```python
from build123d import *

# Parameters (mm, degrees)
SKETCH1_W                   = 355
SKETCH1_H                   = 210
BOSS_EXTRUDE1_DEPTH         = 6
SKETCH2_W                   = 355
SKETCH2_H                   = 92
BOSS_EXTRUDE2_DEPTH         = 7
M4_TAPPED_HOLE2_D           = 3.3
M4_TAPPED_HOLE2_DEPTH       = 2.008579979
M4_TAPPED_HOLE2_CSINK_D     = 4.05
M4_TAPPED_HOLE2_CSINK_ANGLE = 90
M4_TAPPED_HOLE2_TIP         = 0.991420021


with BuildPart() as part:
    # Sketch1 → Boss-Extrude1 (new body)
    with BuildSketch(Plane.XY):
        Rectangle(SKETCH1_W, SKETCH1_H)
    extrude(amount=BOSS_EXTRUDE1_DEPTH)

    # Sketch2 → Boss-Extrude2 (add)
    with BuildSketch(Plane.XY):
        with Locations((0, -59)):
            Rectangle(SKETCH2_W, SKETCH2_H)
    extrude(amount=-BOSS_EXTRUDE2_DEPTH)

    # M4 Tapped Hole2
    with Locations(Plane(origin=(0, 0, -7), x_dir=(-1, 0, 0), z_dir=(0, 0, -1))):
        with Locations((37.5, -29), (-37.5, -29)):
            CounterSinkHole(M4_TAPPED_HOLE2_D / 2, M4_TAPPED_HOLE2_CSINK_D / 2, depth=M4_TAPPED_HOLE2_DEPTH, counter_sink_angle=M4_TAPPED_HOLE2_CSINK_ANGLE)
            with Locations((0, 0, -(M4_TAPPED_HOLE2_DEPTH + M4_TAPPED_HOLE2_TIP / 2))):  # 118° drill point
                Cone(0, M4_TAPPED_HOLE2_D / 2, M4_TAPPED_HOLE2_TIP, mode=Mode.SUBTRACT)


solid = part.part
```
Input: part model. Units: mm. Frame: model coordinates. A direction names the side the tool comes from. Give positions to 0.01 mm unless a question says otherwise; leave off trailing zeros. Order: outer loops, then holes, each group sorted by start corner. A loop starts at its lowest first (then second) coordinate and runs counter-clockwise, first axis right, second up. Notation, with made-up numbers: (65, 5.25) - (107, 5.25) arc R13 cw to (107, 13.25) - close; hole circle Ø3 at (-40, -19). An arc over 180 degrees is marked (long way). One line per item, written item: value.
1. Cut plane A-A, the plane x = -29. Output: boundary loops of the cut face in (y, z), and give its area (3 significant figures).
Determined:
outline: (-105, -7) - (-13, -7) - (-13, 0) - (105, 0) - (105, 6) - (-105, 6) - close
area: 1,900 mm2
2. Line query: probe 1 along X at (y, z) = (-29, -6.2); probe 2 along Y at (x, z) = (37.5, -5.6); probe 3 along Z at (x, y) = (88, 25). Output: solid intervals per line, ascending.
Determined:
probe 1: -177.5 to -39.15, -35.85 to 35.85, 39.15 to 177.5
probe 2: -105 to -30.65, -27.35 to -13
probe 3: 0 to 6
3. Pin query (flat end, axial travel): pin 1 Ø4 at (x, y) = (-37.5, -29) entering from -Z (3 decimals); pin 2 Ø2 at (x, z) = (-34, -3) entering from +Y. Return the tip coordinate at first contact, or that it passes through.
Determined:
pin 1: z = -6.975
pin 2: y = -13
4. Cut plane B-B, the plane y = 20. Output: boundary loops of the cut face in (x, z), and give its area (3 significant figures).
Determined:
outline: (-177.5, 0) - (177.5, 0) - (177.5, 6) - (-177.5, 6) - close
area: 2,130 mm2
5. Reachability of faces 1 (the face through (-2, 1, 6)), 2 (the face through (-2, -13, -3)) from +Z, -Z, +X, -X, +Y, -Y: full face, straight path, thin tool, end or side. Return the list, or none.
Determined:
face 1: +Z, +X, -X, +Y, -Y
face 2: -Z, +X, -X, +Y
